```python
from build123d import *

# Parameters (mm, degrees)
F1_DEPTH = 15
F3_DEPTH = 15
F4_R     = 2
F6_D     = 6.35


with BuildPart() as f1:
    # F0 (on Top) → F1 (new body)
    with BuildSketch(Plane.XY):
        with BuildLine():
            Line((-8, 0), (-25, 0))
            Line((-25, 0), (-25, -2))
            Line((-25, -2), (-8, -2))
            ThreePointArc((-8, -2), (-7.292893, -2.292893), (-7, -3))
            Line((-7, -3), (-7, -5))
            ThreePointArc((-7, -5), (0, -12), (7, -5))
            Line((7, -5), (7, -3))
            ThreePointArc((7, -3), (7.292893, -2.292893), (8, -2))
            Line((8, -2), (25, -2))
            Line((25, -2), (25, 0))
            Line((25, 0), (8, 0))
            ThreePointArc((8, 0), (5.87868, -0.87868), (5, -3))
            Line((5, -3), (5, -5))
            ThreePointArc((5, -5), (0, -10), (-5, -5))
            Line((-5, -5), (-5, -3))
            ThreePointArc((-5, -3), (-5.87868, -0.87868), (-8, 0))
        make_face()
    extrude(amount=F1_DEPTH)

    # F2 (on face) → F3 (join)
    with BuildSketch(Plane.XY.offset(15)):
        with BuildLine():
            Line((-5, -5), (-5, -3))
            ThreePointArc((-5, -3), (-5.87868, -0.87868), (-8, 0))
            Line((-8, 0), (-8, -2))
            ThreePointArc((-8, -2), (-7.292893, -2.292893), (-7, -3))
            Line((-7, -3), (-7, -5))
            ThreePointArc((-7, -5), (0, -12), (7, -5))
            Line((7, -5), (7, -3))
            ThreePointArc((7, -3), (7.292893, -2.292893), (8, -2))
            Line((8, -2), (8, 0))
            ThreePointArc((8, 0), (5.87868, -0.87868), (5, -3))
            Line((5, -3), (5, -5))
            ThreePointArc((5, -5), (0, -10), (-5, -5))
        make_face()
    extrude(amount=F3_DEPTH)

    # F4
    f4_edges = [f1.edges().sort_by_distance(p)[0] for p in [
        (-8, -1, 15),
        (8, -1, 15),
    ]]
    fillet(f4_edges, radius=F4_R)

    # F6 (through all)
    with Locations(Plane(origin=(0, 0, 0), x_dir=(-1, 0, 0), z_dir=(0, 1, 0))):
        with Locations((-17, 7.5), (17, 7.5)):
            Hole(F6_D / 2)


solid = f1.part
```
Design review of the part built by this model. Coordinates are the model's own, in mm. A direction names the side the tool comes from. Give positions to 0.01 mm unless a question says otherwise; leave off trailing zeros. Order: outer loops, then holes, each group sorted by start corner. A loop starts at its lowest first (then second) coordinate and runs counter-clockwise, first axis right, second up. Notation, with made-up numbers: (70.25, 80) -> (96.25, 80) arc R29 cw to (96.25, 109) -> close; hole circle Ø11 at (64.25, -25). An arc over 180 degrees is marked (long way). Write each question's results on one line, items separated by ' | '. Start each with the question number.
Q1. Add section B-B on z = 7.5. Give the boundary of the cut face in (x, y) (3 decimals).
Q2. Mouldability with a two-part tool opening along Z and no side actions: class faces 5 (the flat face through (25, -1, 7)), 6 (the flat face through (-6, -4, 0)), 7 (the flat face through (17, -1, 15)), 8 (the cylindrical face through (-17.69, -1.01, 4.4)) as +Z half, -Z half, draft (parallel to the pull), parting line (faces both ways), or undercut.
Q3. Add section C-C on x = -17. Give the boundary of the cut face in (y, z) (3 decimals).
Q4. For pin 1 (1 mm diameter, centred on y = -1, z = 20.5, fed in from +X); pin 2 (2 mm diameter, centred on y = -4.5, z = 18.5, fed in from +X); pin 3 (1.6 mm diameter, centred on x = -19.5, y = -1.5, fed in from +Z); pin 4 (4 mm diameter, centred on x = -17, z = 7.5, fed in from +Y), all flat-tipped, find the tip position at first contact; note any pin that passes through.
Q5. Add section D-D on z = 27.5. Give the boundary of the cut face in (x, y), and give its area (3 significant figures).
Q6. Add section A-A on y = -4.5. Give the boundary of the cut face in (x, z).
Q7. Wall thickness on L1, parallel to X at y = -3.25, z = 20; L2, parallel to Z at x = 17, y = -0.95 (3 decimals); L3, parallel to Y at x = 0, z = 19.25: over which ranges is each line inside the solid? List them lowest first. Write a range as from..to.
Q8. Machinability: for faces 1 (the flat face through (-7, -4, 15)), 2 (the flat face through (14, -2, 5)), 3 (the cylindrical face through (5.9, -0.86, 14.79)), 4 (the flat face through (-8, -1, 23)), which of the approach directions +Z, -Z, +X, -X, +Y, -Y give a long, thin tool a straight path to every point of the face, cutting with its end or side? Answer none if there is none.
Found:
1) outline: (-25, -2) -> (-20.175, -2) -> (-20.175, 0) -> (-25, 0) -> close; (-13.825, -2) -> (-8, -2) arc R1 cw to (-7, -3) -> (-7, -5) arc R7 ccw to (7, -5) -> (7, -3) arc R1 cw to (8, -2) -> (13.825, -2) -> (13.825, 0) -> (8, 0) arc R3 ccw to (5, -3) -> (5, -5) arc R5 cw to (-5, -5) -> (-5, -3) arc R3 ccw to (-8, 0) -> (-13.825, 0) -> close; (20.175, -2) -> (25, -2) -> (25, 0) -> (20.175, 0) -> close
2) face 5: draft | face 6: -Z half | face 7: +Z half | face 8: undercut
3) outline: (-2, 0) -> (0, 0) -> (0, 4.325) -> (-2, 4.325) -> close; (-2, 10.675) -> (0, 10.675) -> (0, 15) -> (-2, 15) -> close
4) pin 1: stops at x = 8 | pin 2: stops at x = 7 | pin 3: stops at z = 15 | pin 4: passes through
5) outline: (-8, -2) arc R1 cw to (-7, -3) -> (-7, -5) arc R7 ccw to (7, -5) -> (7, -3) arc R1 cw to (8, -2) -> (8, 0) arc R3 ccw to (5, -3) -> (5, -5) arc R5 cw to (-5, -5) -> (-5, -3) arc R3 ccw to (-8, 0) -> close | area: 58.3 mm2
6) outline: (-7, 0) -> (-5, 0) -> (-5, 30) -> (-7, 30) -> close; (5, 0) -> (7, 0) -> (7, 30) -> (5, 30) -> close
7) L1: x = -7..-5, 5..7 | L2: z = 0..4.325, 10.675..15 | L3: y = -12..-10
8) face 1: +Z, -Z, -X, -Y | face 2: +Z, -Z, +X, -Y | face 3: +Z, -Z, +Y | face 4: +Z, -X, +Y, -Y
